Source: three-view drawing plus pictorial views. Frame: mm from the lowest corner of the part. A direction names the side the tool comes from. Give positions to 0.01 mm unless a question says otherwise; leave off trailing zeros. Write each loop counter-clockwise with the first axis right and the second up, starting at its lowest first coordinate (ties: lowest second). Pieces come first, ordered by that corner, then holes. Notation, with made-up numbers: (38.25, 40.5) -> (91.25, 40.5) arc R21 ccw to (91.25, 63.5) -> close; hole circle Ø11 at (-6, 17). An arc over 180 degrees is marked (long way). Answer in a Markdown table with one row per item. Add a question column.
Item 1: Section query A-A on y = 209.55. Output: boundary loops of the cut face in (x, z), plus the area to 3 significant figures.
Item 2: Section query D-D on y = 20. Output: boundary loops of the cut face in (x, z).
Item 3: Material intervals for probe 1 along Y at (x, z) = (37, 6); probe 2 along Z at (x, y) = (44.25, 29.21) (3 decimals); probe 3 along Y at (x, z) = (35.5, 12.7), sorted ascending. Write a range as from..to.
Item 4: First-contact query: P1, Ø2, axis at x = 50.5, z = 22.5, coming from the -Y side; P2, Ø2, axis at y = 155, z = 7, coming from the -X side; P3, Ø7.5, axis at y = 29.21, z = 6.35, coming from the -X side. Flat tips, straight axial feed; report the tip coordinate or a pass-through.
Item 5: Section query C-C on x = 39. Output: boundary loops of the cut face in (y, z) (3 decimals), plus the area to 3 significant figures.
Item 6: Section query B-B on z = 12.7. Output: boundary loops of the cut face in (x, y).
Item 7: Access query for the marked faces 1, 2 and 3. Directions: +Z, -Z, +X, -X, +Y, -Y. A direction counts if a zero-diameter tool reaches every point of the face in a straight line with its end or side. Return the directions, or none.
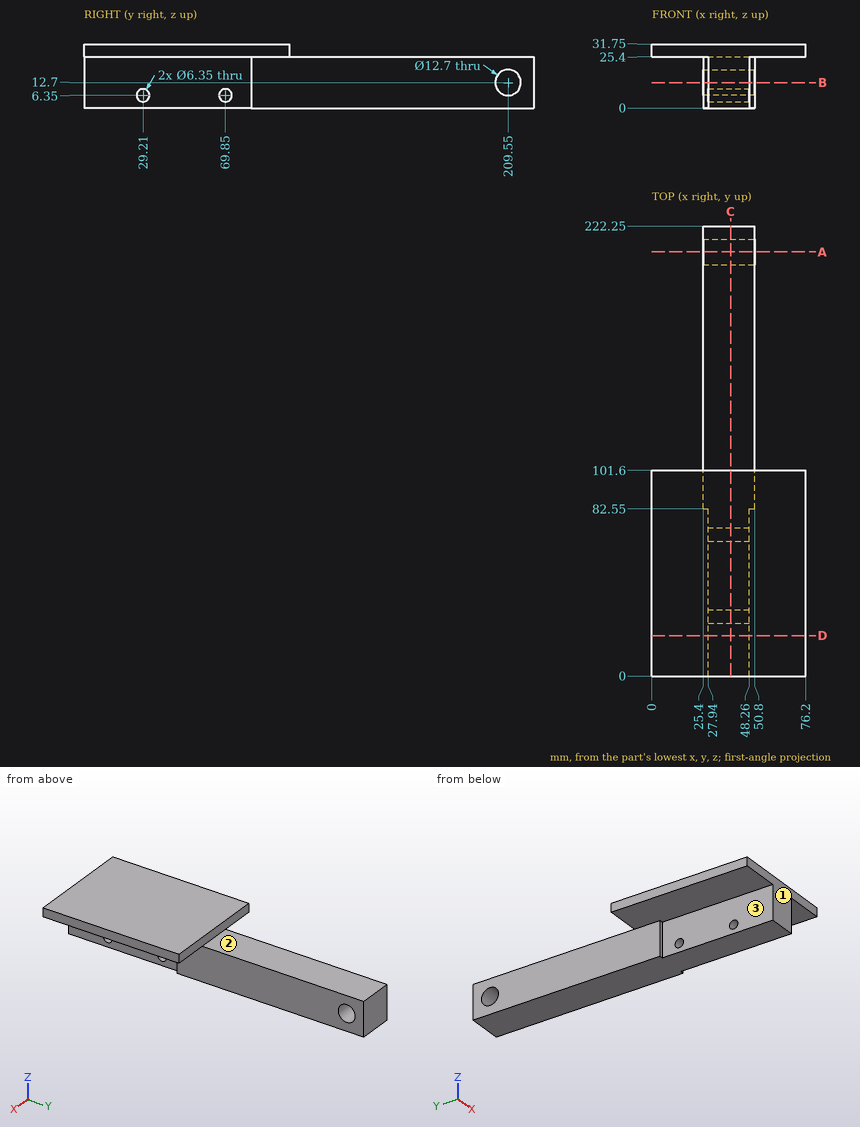
Findings below:
| question | item | result |
|---|---|---|
| 1 | outline | (25.4, 0) -> (50.8, 0) -> (50.8, 6.35) -> (25.4, 6.35) -> close; (25.4, 19.05) -> (50.8, 19.05) -> (50.8, 25.4) -> (25.4, 25.4) -> close |
| 1 | area | 323 mm^2 |
| 2 | outline | (0, 25.4) -> (27.94, 25.4) -> (27.94, 0) -> (48.26, 0) -> (48.26, 25.4) -> (76.2, 25.4) -> (76.2, 31.75) -> (0, 31.75) -> close |
| 3 | probe 1 | y = 0..26.05, 32.37..66.69, 73.01..222.25 |
| 3 | probe 2 | z = 0..3.175, 9.525..31.75 |
| 3 | probe 3 | y = 0..203.2, 215.9..222.25 |
| 4 | P1 | stops at y = 82.55 |
| 4 | P2 | stops at x = 25.4 |
| 4 | P3 | stops at x = 27.94 |
| 5 | outline | (0, 0) -> (222.25, 0) -> (222.25, 25.4) -> (101.6, 25.4) -> (101.6, 31.75) -> (0, 31.75) -> close; hole circle Ø6.35 at (29.21, 6.35); hole circle Ø6.35 at (69.85, 6.35); hole circle Ø12.7 at (209.55, 12.7) |
| 5 | area | 6,100 mm^2 |
| 6 | outline | (25.4, 82.55) -> (27.94, 82.55) -> (27.94, 0) -> (48.26, 0) -> (48.26, 82.55) -> (50.8, 82.55) -> (50.8, 203.2) -> (25.4, 203.2) -> close; (25.4, 215.9) -> (50.8, 215.9) -> (50.8, 222.25) -> (25.4, 222.25) -> close |
| 7 | face 1 | +Z, -Z, +X, -X, -Y |
| 7 | face 2 | +Z, +X, -X, +Y |
| 7 | face 3 | -Z, -X, -Y |
